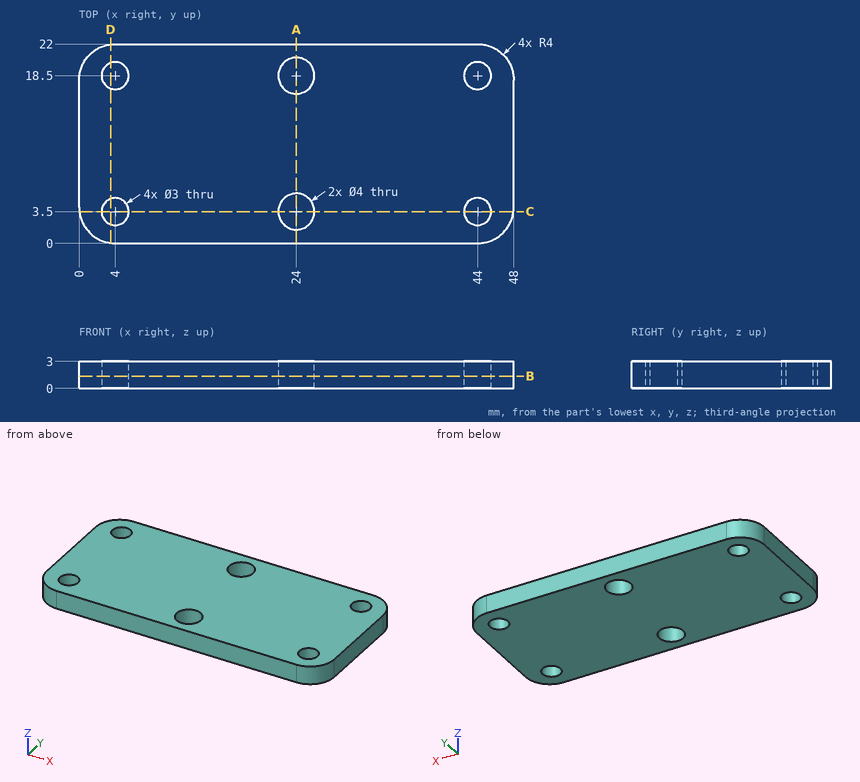
Geometry check sheet. Reference: drawing and pictorial views, mm from the part's lowest x, y, z. Round coordinates to 2 decimals unless told otherwise and drop trailing zeros. Order: outer loops, then holes, each group sorted by start corner. A loop starts at its lowest first (then second) coordinate and runs counter-clockwise, first axis right, second up. Notation, with made-up numbers: (-12.75, 6) - (31.25, 6) arc R18 cw to (31.25, 38) - close; hole circle Ø9 at (11, 0). An arc over 180 degrees is marked (long way). Use a Markdown table: item, result. Add a question column.
1) Section check D-D (x = 3.5). Record the cut outline in (y, z).
2) Section check A-A (x = 24). Record the cut outline in (y, z).
3) Section check C-C (y = 3.5). Record the cut outline in (x, z).
4) Section check B-B (z = 1.35). Record the cut outline in (x, y).
5) Gauge pin test, flat ends, axial feed: P1, Ø4, axis at x = 44, y = 18.5, coming from the +Z side; P2, Ø3.5, axis at x = 24, y = 18.5, coming from the +Z side. Record the tip position at first contact, or that the pin passes through.
6) Thickness scan on line 1 along Y through (x, z) = (24, 2.3); line 2 along Y through (x, z) = (44, 2.2); line 3 along X through (y, z) = (17.25, 1.65). Record the ranges inside material, lowest first.
Established:
| question | item | result |
|---|---|---|
| 1 | outline | (0.03, 0) - (2.09, 0) - (2.09, 3) - (0.03, 3) - close; (4.91, 0) - (17.09, 0) - (17.09, 3) - (4.91, 3) - close; (19.91, 0) - (21.97, 0) - (21.97, 3) - (19.91, 3) - close |
| 2 | outline | (0, 0) - (1.5, 0) - (1.5, 3) - (0, 3) - close; (5.5, 0) - (16.5, 0) - (16.5, 3) - (5.5, 3) - close; (20.5, 0) - (22, 0) - (22, 3) - (20.5, 3) - close |
| 3 | outline | (0.03, 0) - (2.5, 0) - (2.5, 3) - (0.03, 3) - close; (5.5, 0) - (22, 0) - (22, 3) - (5.5, 3) - close; (26, 0) - (42.5, 0) - (42.5, 3) - (26, 3) - close; (45.5, 0) - (47.97, 0) - (47.97, 3) - (45.5, 3) - close |
| 4 | outline | (0, 4) arc R4 ccw to (4, 0) - (44, 0) arc R4 ccw to (48, 4) - (48, 18) arc R4 ccw to (44, 22) - (4, 22) arc R4 ccw to (0, 18) - close; hole circle Ø3 at (4, 3.5); hole circle Ø3 at (4, 18.5); hole circle Ø4 at (24, 3.5); hole circle Ø4 at (24, 18.5); hole circle Ø3 at (44, 3.5); hole circle Ø3 at (44, 18.5) |
| 5 | P1 | z = 3 |
| 5 | P2 | through |
| 6 | line 1 | 0 to 1.5, 5.5 to 16.5, 20.5 to 22 |
| 6 | line 2 | 0 to 2, 5 to 17, 20 to 22 |
| 6 | line 3 | 0 to 3.17, 4.83 to 22.44, 25.56 to 43.17, 44.83 to 48 |
